from build123d import *
from build123d import SkipClean  # not in build123d's __all__

# Parameters (mm, degrees)
F0_R      = 9
F0_W      = 39.5156368613
F0_H      = 4.7
F0_W_2    = 39.887715684
F0_R_2    = 10
F1_DEPTH  = 2.5
F2_R      = 1.4160019586
F3_R      = 4.1166770091
F4_R      = 2.0561745665
F5_R      = 5
F6_R      = 1.5425858978
F7_R      = 5
F8_R      = 5
F10_R     = 1.5
F11_DEPTH = 25


with BuildPart() as f1:
    # F0 (on Top) → F1 (new body)
    with BuildSketch(Plane.XY):
        with BuildLine():
            Line((74.8763903975, -38.2511245025), (69.3773250177, -38.2511245025))
            ThreePointArc((69.3773250177, -38.2511245025), (67.8773250177, -39.7511245025), (66.3773250177, -38.2511245025))
            Line((66.3773250177, -38.2511245025), (62.3773250177, -38.2511245025))
            ThreePointArc((62.3773250177, -38.2511245025), (60.8773250177, -39.7511245025), (59.3773250177, -38.2511245025))
            Line((59.3773250177, -38.2511245025), (55.3773250177, -38.2511245025))
            ThreePointArc((55.3773250177, -38.2511245025), (53.8773250177, -39.7511245025), (52.3773250177, -38.2511245025))
            Line((52.3773250177, -38.2511245025), (48.3773250177, -38.2511245025))
            ThreePointArc((48.3773250177, -38.2511245025), (46.8773250177, -39.7511245025), (45.3773250177, -38.2511245025))
            Line((45.3773250177, -38.2511245025), (41.3773250177, -38.2511245025))
            ThreePointArc((41.3773250177, -38.2511245025), (39.8773250177, -39.7511245025), (38.3773250177, -38.2511245025))
            Line((38.3773250177, -38.2511245025), (34.3773250177, -38.2511245025))
            ThreePointArc((34.3773250177, -38.2511245025), (32.8773250177, -39.7511245025), (31.3773250177, -38.2511245025))
            Line((31.3773250177, -38.2511245025), (-66.1923438311, -38.2511245025))
            Line((-66.1923438311, -38.2511245025), (-66.1923438311, -66.2511245025))
            Line((-66.1923438311, -66.2511245025), (-81.1216448216, -80.6109128623))
            Line((-81.1216448216, -80.6109128623), (-81.1216448216, -113.3109128623))
            Line((-81.1216448216, -113.3109128623), (-73.3216448216, -113.3109128623))
            Line((-73.3216448216, -113.3109128623), (-73.3216448216, -117.8109128623))
            Line((-73.3216448216, -117.8109128623), (-81.1216448216, -117.8109128623))
            Line((-81.1216448216, -117.8109128623), (-81.1216448216, -125.6109128623))
            Line((-81.1216448216, -125.6109128623), (-56.1216448216, -125.6109128623))
            Line((-56.1216448216, -125.6109128623), (-35.532054749, -106.3894852996))
            Line((-35.532054749, -106.3894852996), (-35.532054749, -87.3894852996))
            Line((-35.532054749, -87.3894852996), (38.0006051308, -87.3894852996))
            Line((38.0006051308, -87.3894852996), (46.9109937549, -82.7472803621))
            Line((46.9109937549, -82.7472803621), (46.9109937549, -78.8513062))
            Line((46.9109937549, -78.8513062), (60.7595592737, -78.8513062))
            Line((60.7595592737, -78.8513062), (60.7595592737, -83.155875459))
            Line((60.7595592737, -83.155875459), (76.8783551784, -78.677393496))
            Line((76.8783551784, -78.677393496), (76.8783551784, -51.0392449796))
            Line((76.8783551784, -51.0392449796), (74.8763903975, -43.6687730253))
            Line((74.8763903975, -43.6687730253), (74.8763903975, -38.2511245025))
        make_face()
        with Locations((-63.9078766108, -103.1785532832)):
            Circle(F0_R, mode=Mode.SUBTRACT)
        with Locations((-27.756717056, -78.7394852996)):
            Rectangle(F0_W, F0_H, mode=Mode.SUBTRACT)
        with Locations((-27.756717056, -70.2394852996)):
            Rectangle(F0_W, F0_H, mode=Mode.SUBTRACT)
        with Locations((20.3393899865, -78.7394852996)):
            Rectangle(F0_W_2, F0_H, mode=Mode.SUBTRACT)
        with Locations((20.3393899865, -70.2394852996)):
            Rectangle(F0_W_2, F0_H, mode=Mode.SUBTRACT)
        with Locations((59.0378009468, -62.0803784949)):
            Circle(F0_R_2, mode=Mode.SUBTRACT)
    extrude(amount=F1_DEPTH)

    # F2
    f2_edges = [f1.edges().sort_by_distance(p)[0] for p in [
        (60.759559, -83.155875, 1.25),
    ]]
    fillet(f2_edges, radius=F2_R)

    # F3
    f3_edges = [f1.edges().sort_by_distance(p)[0] for p in [
        (76.878355, -78.677393, 1.25),
    ]]
    fillet(f3_edges, radius=F3_R)

    # F4
    f4_edges = [f1.edges().sort_by_distance(p)[0] for p in [
        (46.910994, -82.74728, 1.25),
        (38.000605, -87.389485, 1.25),
    ]]
    fillet(f4_edges, radius=F4_R)

    # F5
    f5_edges = [f1.edges().sort_by_distance(p)[0] for p in [
        (-56.121645, -125.610913, 1.25),
        (-35.532055, -106.389485, 1.25),
    ]]
    fillet(f5_edges, radius=F5_R)

    # F6
    f6_edges = [f1.edges().sort_by_distance(p)[0] for p in [
        (-81.121645, -113.310913, 1.25),
        (-81.121645, -117.810913, 1.25),
        (-81.121645, -125.610913, 1.25),
    ]]
    fillet(f6_edges, radius=F6_R)

    # F7
    f7_edges = [f1.edges().sort_by_distance(p)[0] for p in [
        (-81.121645, -80.610913, 1.25),
        (-66.192344, -66.251125, 1.25),
    ]]
    fillet(f7_edges, radius=F7_R)

    # F8
    f8_edges = [f1.edges().sort_by_distance(p)[0] for p in [
        (76.878355, -51.039245, 1.25),
        (74.87639, -43.668773, 1.25),
    ]]
    fillet(f8_edges, radius=F8_R)

    # F9: F1 across face


with BuildPart() as f1_1:
    add(f1.part, clean=False)
    with SkipClean():  # cleaning this boolean's faces spoils the solid; the shape is the same uncleaned
        add(f1.part.mirror(Plane(origin=(-17.4075094067, -38.2511245025, 1.25), x_dir=(-1, 0, 0), z_dir=(0, 1, 0))), clean=False)

    # F10 (on face) → F11 (cut)
    with BuildSketch(Plane.XY.offset(2.5)):
        with Locations((-59.1923438311, -18.2511245025)):
            Circle(F10_R)
        with Locations((-18.1923438311, -18.2511245025)):
            Circle(F10_R)
        with Locations((-18.1923438311, -58.2511245025)):
            Circle(F10_R)
        with Locations((-59.1923438311, -58.2511245025)):
            Circle(F10_R)
        with Locations((3.8763903975, -18.2511245025)):
            Circle(F10_R)
        with Locations((3.8763903975, -58.2511245025)):
            Circle(F10_R)
        with Locations((44.8763903975, -58.2511245025)):
            Circle(F10_R)
        with Locations((44.8763903975, -18.2511245025)):
            Circle(F10_R)
    extrude(amount=-F11_DEPTH, mode=Mode.SUBTRACT)


solid = f1_1.part
Design review of the part built by this model. Coordinates are the model's own, in mm. A direction names the side the tool comes from. Coordinates: 2 decimals unless noted, no trailing zeros. Order: outer loops, then holes, each group sorted by start corner. A loop starts at its lowest first (then second) coordinate and runs counter-clockwise, first axis right, second up. Notation, with made-up numbers: (79, 88) - (118, 88) arc R28 cw to (118, 124) - close; hole circle Ø8 at (12.5, 9.25). An arc over 180 degrees is marked (long way). Put each result on its own line as item: value.
1) Take a section at B-B, the plane z = 0.7. Count the separate pieces of the cut face and the enclosed holes in it, and give its area (3 significant figures).
Response values:
separate pieces: 1
enclosed holes: 26
area: 14,200 mm²
2) The part is to be moulded in two halves that separate along Y. For faces 3 (the face through (-3, -39, 0)), 4 (the face through (-46.02, -116.18, 1.23)), 5 (the face through (-73.574, -3.151, 1.232)), 6 (the face through (-46.02, 39.68, 1.23)), say which applies: released by +Y, released by -Y, zero draft, split by the parting line, or undercut.
Response values:
face 3: zero draft
face 4: released by -Y
face 5: undercut
face 6: released by +Y
3) Wall thickness on L1, parallel to Y at x = 23, z = 1.55; L2, parallel to Y at x = -70, z = 1.7; L3, parallel to X at y = -15, z = 1.35: over which ranges is each line inside the solid? List them lowest first. Write a range as from..to.
Response values:
L1: y = -87.39..-81.09, -76.39..-72.59, -67.89..-8.61, -3.91..-0.11, 4.59..10.89
L2: y = -125.61..-109.8, -96.55..-69.91, -6.59..20.05, 33.3..49.11
L3: x = -66.19..49.05, 69.02..76.88
4) Insertion check: P1, Ø2.5, axis at x = -59.19, y = -18.25, coming from the -Z side; P2, Ø1.2, axis at y = 3, z = 1, coming from the -X side; P3, Ø1.2, axis at x = -19.5, z = 1, coming from the -Y side; P4, Ø1.2, axis at x = 21, z = 1, coming from the +Y side. Each pin has a flat end and moves straight along its axis. Give the tip position at first contact, or say it passes through.
Response values:
P1: passes through
P2: stops at x = -80.37
P3: stops at y = -87.39
P4: stops at y = 10.89
5) Tool access review of faces 1 (the face through (-65.859, -111.965, 1.232)), 2 (the face through (-73.57, -73.35, 1.23)): name each direction out of +Z, -Z, +X, -X, +Y, -Y from which nothing blocks a thin tool from reaching the whole face with its end or side.
Response values:
face 1: +Z, -Z
face 2: +Z, -Z, -X
6) Take a section at A-A, the plane x = 27.5. Give the boundary of the cut face in (y, z), and give its area (3 significant figures).
Response values:
outline: (-87.39, 0) - (-81.09, 0) - (-81.09, 2.5) - (-87.39, 2.5) - close; (-76.39, 0) - (-72.59, 0) - (-72.59, 2.5) - (-76.39, 2.5) - close; (-67.89, 0) - (-8.61, 0) - (-8.61, 2.5) - (-67.89, 2.5) - close; (-3.91, 0) - (-0.11, 0) - (-0.11, 2.5) - (-3.91, 2.5) - close; (4.59, 0) - (10.89, 0) - (10.89, 2.5) - (4.59, 2.5) - close
area: 199 mm²
